Check sheet for the modelled part. Datum: model origin and axes. Units: mm. Face numbers are marked on the shaded views. A direction names the side the tool comes from. Round coordinates to 2 decimals unless told otherwise and drop trailing zeros. Write each loop counter-clockwise with the first axis right and the second up, starting at its lowest first coordinate (ties: lowest second). Pieces come first, ordered by that corner, then holes. Notation, with made-up numbers: (7.5, 61.25) -> (13.5, 61.25) arc R30 cw to (13.5, 94.25) -> close; hole circle Ø10 at (-22.5, -23). An arc over 180 degrees is marked (long way). One line per item, written item: value.
Autodesk Inventor part; units mm, degrees
ref_plane "YZ Plane" through (0, 0, 0) normal (1, 0, 0) x (0, 1, 0)
ref_plane "XZ Plane" through (0, 0, 0) normal (0, 1, 0) x (-1, 0, 0)
ref_plane "XY Plane" through (0, 0, 0) normal (0, 0, 1) x (1, 0, 0)
sketch "Sketch1" plane through (0, 0, 0) normal (0, 0, 1) x (1, 0, 0)
  arc A0 (34.5919, 154.5766) -> (21.7257, 156.9029) centre (0, 0) ccw
  line L0 (38.5, 149.6973) -> (38.5, 147.1504)
  line L1 (-38.5, 147.1504) -> (-38.5, 149.6973)
  arc A1 (18.2237, 161.8774) -> (-18.2237, 161.8774) centre (0, 0) ccw
  line L2 (20, 159.8899) -> (20, 158.884)
  line L3 (-20, 158.884) -> (-20, 159.8899)
  arc A2 (-21.7257, 156.9029) -> (-34.5919, 154.5766) centre (0, 0) ccw
  arc A3 (32.3901, 142.2751) -> (20.1378, 144.5192) centre (0, 0) ccw
  arc A4 (-20.1378, 144.5192) -> (-32.3901, 142.2751) centre (0, 0) ccw
  line L4 (-19.8618, 144.5384) -> (19.8618, 144.5384)
  arc A5 (-38.5, 147.1504) -> (-32.3901, 142.2751) centre (-33.5, 147.1504) ccw
  arc A6 (-34.5919, 154.5766) -> (-38.5, 149.6973) centre (-33.5, 149.6973) ccw
  arc A7 (32.3901, 142.2751) -> (38.5, 147.1504) centre (33.5, 147.1504) ccw
  arc A8 (38.5, 149.6973) -> (34.5919, 154.5766) centre (33.5, 149.6973) ccw
  arc A9 (-21.7257, 156.9029) -> (-20, 158.884) centre (-22, 158.884) ccw
  arc A10 (20, 158.884) -> (21.7257, 156.9029) centre (22, 158.884) ccw
  arc A11 (20, 159.8899) -> (18.2237, 161.8774) centre (18, 159.8899) ccw
  arc A12 (-18.2237, 161.8774) -> (-20, 159.8899) centre (-18, 159.8899) ccw
  arc A13 (-19.8618, 144.5384) -> (-20.1378, 144.5192) centre (-19.8618, 142.5384) ccw
  arc A14 (20.1378, 144.5192) -> (19.8618, 144.5384) centre (19.8618, 142.5384) ccw
  point P0 (38.5, 140.7448)
  point P1 (38.5, 153.6499)
  point P2 (-38.5, 140.7448)
  point P3 (-38.5, 153.6499)
  point P4 (20, 161.6675)
  point P5 (20, 144.5384)
  point P6 (-20, 144.5384)
  point P7 (-20, 161.6675)
  point P8 (-20, 157.1322)
  point P9 (20, 157.1322)
  dimension "d5" = 77
  dimension "d6" = 38.5
  dimension "d9" = 5
  dimension "d10" = 2
extrude "Extrusion1" add sketch "Sketch1" along normal blind 5
sketch "Sketch2" plane through (0, 0, 5) normal (0, 0, 1) x (1, 0, 0)
  line L0 (-19, 145.5384) -> (19, 145.5384)
  line L1 (19, 145.5384) -> (19, 160.5384)
  line L2 (19, 160.5384) -> (-19, 160.5384)
  line L3 (-19, 160.5384) -> (-19, 145.5384)
  circle A0 centre (-31, 149.5384) radius 1.5
  circle A1 centre (-25, 151.0384) radius 1.5
  line L4 (-19.8618, 144.5384) -> (19.8618, 144.5384)
  point P0 (0, 0)
  point P1 (0, 145.5384)
  point P2 (0, 144.5384)
  dimension "d13" = 38
  dimension "d14" = 15
  dimension "d15" = 1
  dimension "d16" = 25
  dimension "d17" = 31
  dimension "d18" = 3
  dimension "d19" = 3
  dimension "d20" = 5
  dimension "d21" = 1.5
extrude "Extrusion2" add sketch "Sketch2" along normal blind 4 contours L3 L2 L1 L0
hole "Hole1" at (-31, 149.5384, 5) at (-25, 151.0384, 5) direction (0, 0, -1) diameter 3 end through all countersink diameter 6 countersink angle 90
mirror "Mirror1" about plane through (0, 0, 0) normal (1, 0, 0) of "Hole1"
fillet "Fillet1" radius 2 4 edges at (0, 160.5384, 9) (-19, 153.0384, 9) (0, 145.5384, 9) (19, 153.0384, 9)
equation "\"d19\" = d18"
properties part number "magnet" material "Iron, Gray"
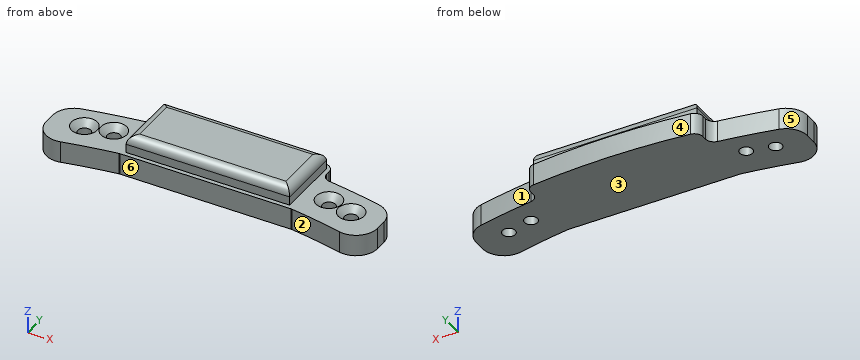
Item 1: Sectioned sample at C-C on y = 151.75. Count the separate pieces of the cut face and the enclosed holes in it, and give its area (3 significant figures).
Answer:
separate pieces: 3
enclosed holes: 0
area: 495 mm^2
Item 2: Thickness scan on line 1 (X direction, y = 151.25, z = 4.5); line 2 (X direction, y = 150.5, z = 1); line 3 (Z direction, x = -28, y = 146.75). Record the ranges inside material, lowest first.
Answer:
line 1: x = -38.25 to -32.82, -29.18 to -27.49, -22.51 to 22.51, 27.49 to 29.18, 32.82 to 38.25
line 2: x = -38.44 to -32.15, -29.85 to -26.4, -23.6 to 23.6, 26.4 to 29.85, 32.15 to 38.44
line 3: z = 0 to 5
Item 3: Sectioned sample at A-A on x = 25. Enter the section's corners in (y, z), and give its area (3 significant figures).
Answer:
outline: (143.76, 0) -> (149.54, 0) -> (149.54, 3.5) -> (148.04, 5) -> (143.76, 5) -> close; (152.54, 0) -> (156.41, 0) -> (156.41, 5) -> (154.04, 5) -> (152.54, 3.5) -> close
area: 46.0 mm^2
Item 4: Tool access check on the marked faces 5 and 6. Record the directions out of +Z, -Z, +X, -X, +Y, -Y that give a thin tool (end or side, any length) a straight path to the whole face; none if there is none.
Answer:
face 5: +Z, -Z, -X, +Y
face 6: +Z, -Z, -Y
Item 5: Depth check by flat-ended pin: P1, Ø1, axis at y = 156, z = 6.5, coming from the -X side; P2, Ø2, axis at x = 21.5, z = 8, coming from the -Y side; P3, Ø2.5, axis at x = -6, z = 2.5, coming from the -Y side; P4, Ø1.1, axis at y = 159.5, z = 2, coming from the +X side. Enter the tip coordinate at first touch or a pass-through.
Answer:
P1: stops at x = -19
P2: passes through
P3: stops at y = 144.54
P4: stops at x = 20
Item 6: Mould release check, pull along X, two halves, no side actions. Record for the marked faces 1, 2, 3 and 4: pulls with the +X half, pulls with the -X half, needs draft (parallel to the pull), parting line crosses it, or undercut.
Answer:
face 1: pulls with the +X half
face 2: undercut
face 3: needs draft
face 4: parting line crosses it
Item 7: Sectioned sample at B-B on x = -7. Enter the section's corners in (y, z).
Answer:
outline: (144.54, 0) -> (162.75, 0) -> (162.75, 5) -> (160.54, 5) -> (160.54, 7) arc R2 ccw to (158.54, 9) -> (147.54, 9) arc R2 ccw to (145.54, 7) -> (145.54, 5) -> (144.54, 5) -> close
Item 8: Sectioned sample at D-D on z = 5.75. Enter the section's corners in (x, y), and give its area (3 significant figures).
Answer:
outline: (-19, 145.54) -> (19, 145.54) -> (19, 160.54) -> (-19, 160.54) -> close
area: 570 mm^2
